Geometry: see drawing. Coordinates: mm, zero at the bounding-box minimum. A direction names the side the tool comes from. Give positions to 0.01 mm unless a question says otherwise; leave off trailing zeros. Order: outer loops, then holes, each group sorted by start corner. A loop starts at its lowest first (then second) coordinate and runs counter-clockwise, first axis right, second up. Notation, with made-up numbers: (-16, 23) - (2, 23) arc R14 ccw to (2, 27) - close; hole circle Ø5 at (46, 37). An arc over 180 degrees is marked (long way). One line per item, written item: value.
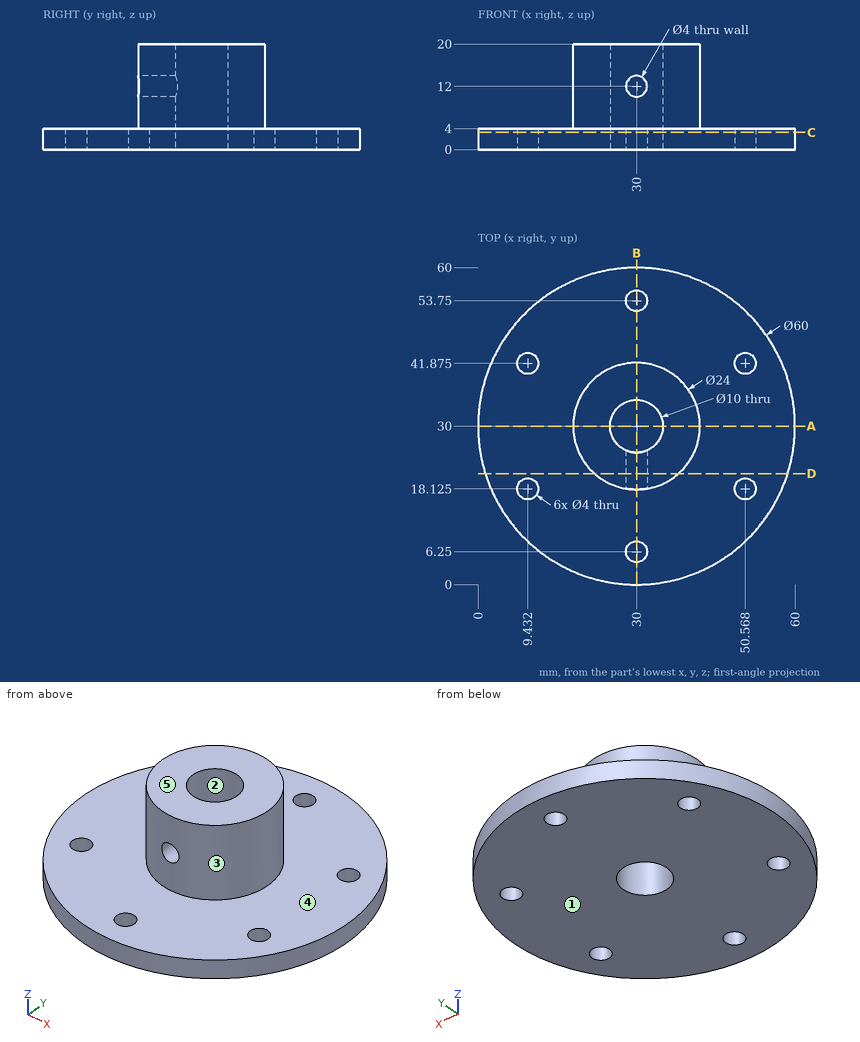
1) Set-up query: the marked faces 4 and 5. Return all of +Z, -Z, +X, -X, +Y, -Y with unobstructed straight access to the full face (end or side cutting, diameter ignored); none if empty.
Answers below:
face 4: +Z
face 5: +Z, +X, -X, +Y, -Y
2) Section C-C, the plane z = 3.25. Return loops of the section in (x, y) (3 decimals), then the cut area to 3 significant figures.
Answers below:
outline: circle Ø60 at (30, 30); hole circle Ø4 at (9.432, 18.125); hole circle Ø4 at (9.432, 41.875); hole circle Ø10 at (30, 30); hole circle Ø4 at (30, 6.25); hole circle Ø4 at (30, 53.75); hole circle Ø4 at (50.568, 18.125); hole circle Ø4 at (50.568, 41.875)
area: 2,670 mm^2
3) Material intervals for line 1 along Z through (x, y) = (30, 23); line 2 along Y through (x, z) = (8.5, 1.25) (1 decimal); line 3 along Y through (x, z) = (30, 11.25), sorted ascending.
Answers below:
line 1: 0 to 10, 14 to 20
line 2: 9.1 to 16.4, 19.9 to 40.1, 43.6 to 50.9
line 3: 35 to 42
4) Section D-D, the plane y = 21. Return loops of the section in (x, z), then the cut area to 3 significant figures.
Answers below:
outline: (1.38, 0) - (58.62, 0) - (58.62, 4) - (37.94, 4) - (37.94, 20) - (22.06, 20) - (22.06, 4) - (1.38, 4) - close; hole circle Ø4 at (30, 12)
area: 470 mm^2
5) First-contact query: pin 1 (3.5 mm diameter, centred on x = 30, z = 12, fed in from +Y); pin 2 (9 mm diameter, centred on x = 30, y = 30, fed in from +Z); pin 3 (4 mm diameter, centred on y = 41.5, z = 15.5, fed in from -X); pin 4 (12 mm diameter, centred on y = 25, z = 15, fed in from +X). Flat tips, straight axial feed; report the tip coordinate or a pass-through.
Answers below:
pin 1: y = 42
pin 2: through
pin 3: x = 22.67
pin 4: x = 42
6) Mould query, pull axis X, two halves, no side actions, for the marked faces 1, 2 and 3. Classes: released by +X, released by -X, zero draft, split by the parting line, or undercut.
Answers below:
face 1: zero draft
face 2: undercut
face 3: split by the parting line
7) Section B-B, the plane x = 30. Return loops of the section in (y, z).
Answers below:
outline: (0, 0) - (4.25, 0) - (4.25, 4) - (0, 4) - close; (8.25, 0) - (25, 0) - (25, 10) - (18, 10) - (18, 4) - (8.25, 4) - close; (18, 14) - (25, 14) - (25, 20) - (18, 20) - close; (35, 0) - (51.75, 0) - (51.75, 4) - (42, 4) - (42, 20) - (35, 20) - close; (55.75, 0) - (60, 0) - (60, 4) - (55.75, 4) - close
8) Section A-A, the plane y = 30. Return loops of the section in (x, z).
Answers below:
outline: (0, 0) - (25, 0) - (25, 20) - (18, 20) - (18, 4) - (0, 4) - close; (35, 0) - (60, 0) - (60, 4) - (42, 4) - (42, 20) - (35, 20) - close
